The model under review builds one solid part; all positions refer to its coordinate system, in mm. A direction names the side the tool comes from. Round coordinates to 2 decimals unless told otherwise and drop trailing zeros. Order: outer loops, then holes, each group sorted by start corner. A loop starts at its lowest first (then second) coordinate and runs counter-clockwise, first axis right, second up.
from build123d import *

# Parameters (mm, degrees)
SKETCH1_R               = 4
BOSS_EXTRUDE1_DEPTH     = 40
FILLET1_R               = 5
SKETCH2_W               = 25
SKETCH2_H               = 25
CUT_EXTRUDE1_DEPTH      = 9
CUT_EXTRUDE1_DEPTH_BACK = 52.87
FILLET2_R               = 2


with BuildPart() as part:
    # Sketch1 → Boss-Extrude1 (new body)
    with BuildSketch(Plane.XY):
        with BuildLine():
            Line((6.947546174, -51.87), (-7.673645346, -2.261673518))
            ThreePointArc((-7.673645346, -2.261673518), (-5.46693216, 5.840603801), (2.763356291, 7.507586963))
            Line((2.763356291, 7.507586963), (123.33, -36.87))
            Line((123.33, -36.87), (127.33, -51.87))
            Line((127.33, -51.87), (101.494792958, -51.87))
            ThreePointArc((101.494792958, -51.87), (70.04, -38.09), (38.585207042, -51.87))
            Line((38.585207042, -51.87), (6.947546174, -51.87))
        make_face()
        Circle(SKETCH1_R, mode=Mode.SUBTRACT)
        with Locations((7.33, -24.87)):
            Circle(SKETCH1_R, mode=Mode.SUBTRACT)
    extrude(amount=-BOSS_EXTRUDE1_DEPTH)

    # Fillet1
    fillet1_edges = [part.edges().sort_by_distance(p)[0] for p in [
        (6.947546174, -51.87, -20),
        (123.33, -36.87, -20),
        (127.33, -51.87, -20),
    ]]
    fillet(fillet1_edges, radius=FILLET1_R)

    # Sketch2 → Cut-Extrude1 (cut, two sides)
    with BuildSketch(Plane(origin=(0, 0, 0), x_dir=(1, 0, 0), z_dir=(0, 1, 0))) as cut_extrude1_sk:
        with Locations((2.5, 20)):
            Rectangle(SKETCH2_W, SKETCH2_H)
    extrude(amount=CUT_EXTRUDE1_DEPTH, mode=Mode.SUBTRACT)
    extrude(cut_extrude1_sk.sketch, amount=-CUT_EXTRUDE1_DEPTH_BACK, mode=Mode.SUBTRACT)

    # Fillet2
    fillet2_edges = [part.edges().sort_by_distance(p)[0] for p in [
        (15, -24.433208829, -7.5),
        (15, -24.433208829, -32.5),
    ]]
    fillet(fillet2_edges, radius=FILLET2_R)


solid = part.part
(1) We need section D-D (z = -22). Give the boundary of the cut face in (x, y), and give its area (3 significant figures).
(2) We need section B-B (y = -24.87). Give the boundary of the cut face in (x, z).
(3) To check wall thickness, follow L1, parallel to Z at x = 6, y = -32; L2, parallel to Y at x = 7.33, z = -3.75; L3, parallel to Y at x = 96, z = -22. State the ranges of each line that lie inside material, in increasing order.
(4) The part is to be moulded in two halves that separate along Y. For faces 3 (the cylindrical face through (7.66, -50.85, -3.8)), 4 (the cylindrical face through (-0.867, -3.905, -36.198)), 5 (the flat face through (15, -24, -20)), say which applies: pulls with the +Y half, pulls with the -Y half, needs draft (parallel to the pull), parting line crosses it, or undercut.
(5) Tool access review of faces 1 (the flat face through (-0.8, -25.59, -3.7)), 2 (the flat face through (5, -15, -32.5)): name each direction out of +Z, -Z, +X, -X, +Y, -Y from which nothing blocks a thin tool from reaching the whole face with its end or side.
(6) We need section A-A (z = -35.5). Give the boundary of the cut face in (x, y), and give its area (3 significant figures).
(7) Clearance check with flat-ended pins moving along their axes: P1, Ø1.5, axis at y = -26, z = -6.5, coming from the -X side; P2, Ø5, axis at x = 7.33, y = -24.87, coming from the -Z side; P3, Ø10.5, axis at x = 5.5, y = -18, coming from the +Z side; P4, Ø8, axis at x = 78, z = -34.5, coming from the +Y side. State where each tip first meets the part, or that it passes through.
(8) We need section C-C (x = 0). Give the boundary of the cut face in (y, z).
Verdict:
1. outline: (15, -51.87) - (38.59, -51.87) arc R42.79 cw to (101.49, -51.87) - (120.82, -51.87) arc R5 ccw to (125.65, -45.58) - (124, -39.38) arc R5 ccw to (120.89, -35.97) - (15, 3) - close
1. area: 3,200 mm2
2. outline: (-1.01, -40) - (3.33, -40) - (3.33, -32.5) - (-1.01, -32.5) - close; (-1.01, -7.5) - (3.33, -7.5) - (3.33, 0) - (-1.01, 0) - close; (11.33, -40) - (90.73, -40) - (90.73, 0) - (11.33, 0) - (11.33, -7.5) - (13, -7.5) arc R2 cw to (15, -9.5) - (15, -30.5) arc R2 cw to (13, -32.5) - (11.33, -32.5) - close
3. L1: z = -40 to -32.5, -7.5 to 0
3. L2: y = -50.58 to -28.87, -20.87 to 5.83
3. L3: y = -46.86 to -26.81
4. face 3: pulls with the -Y half
4. face 4: undercut
4. face 5: needs draft
5. face 1: +Z, -Z, -X, -Y
5. face 2: -X, +Y, -Y
6. outline: (-7.67, -2.26) - (5.89, -48.28) arc R5 ccw to (10.69, -51.87) - (38.59, -51.87) arc R42.79 cw to (101.49, -51.87) - (120.82, -51.87) arc R5 ccw to (125.65, -45.58) - (124, -39.38) arc R5 ccw to (120.89, -35.97) - (2.76, 7.51) arc R8 ccw to start; hole circle Ø8 at (0, 0); hole circle Ø8 at (7.33, -24.87)
6. area: 4,050 mm2
7. P1: stops at x = -0.9
7. P2: passes through
7. P3: stops at z = 0
7. P4: stops at y = -18.71
8. outline: (-28.3, -40) - (-4, -40) - (-4, -32.5) - (-28.3, -32.5) - close; (-28.3, -7.5) - (-4, -7.5) - (-4, 0) - (-28.3, 0) - close; (4, -40) - (8, -40) - (8, -32.5) - (4, -32.5) - close; (4, -7.5) - (8, -7.5) - (8, 0) - (4, 0) - close
